```python
from build123d import *

# Parameters (mm, degrees)
SALIENTE_EXTRUIR1_DEPTH = 300
VACIADO1_START          = 47.215476502
VACIADO1_DEPTH          = 295
CROQUIS3_R              = 7.5
CROQUIS3_R_2            = 10
CROQUIS3_W              = 35.4
CROQUIS3_H              = 33.7
CORTAR_EXTRUIR1_DEPTH   = 15
SALIENTE_EXTRUIR2_START = -150
SALIENTE_EXTRUIR2_DEPTH = 150
VACIADO3_START          = 197.215476502
VACIADO3_DEPTH          = 145
CROQUIS5_W              = 5
CROQUIS5_H              = 70
SALIENTE_EXTRUIR3_DEPTH = 145
CROQUIS6_R              = 12.5
CORTAR_EXTRUIR2_DEPTH   = 15
CROQUIS7_W              = 210
CROQUIS7_H              = 255
CORTAR_EXTRUIR3_DEPTH   = 5
SALIENTE_EXTRUIR4_DEPTH = 70
SALIENTE_EXTRUIR5_START = -150
SALIENTE_EXTRUIR5_DEPTH = 150
CORTAR_EXTRUIR6_START   = -150
CORTAR_EXTRUIR6_DEPTH   = 150
CORTAR_EXTRUIR7_START   = -150
CORTAR_EXTRUIR7_DEPTH   = 150
CORTAR_EXTRUIR9_DEPTH   = 15
CROQUIS19_R             = 5
CORTAR_EXTRUIR10_DEPTH  = 15
SALIENTE_EXTRUIR6_START = -5
SALIENTE_EXTRUIR6_DEPTH = 5
CROQUIS21_W             = 25
CROQUIS21_H             = 25
CROQUIS21_R             = 5
SALIENTE_EXTRUIR7_DEPTH = 7
CROQUIS22_R             = 5
CORTAR_EXTRUIR13_DEPTH  = 7
CROQUIS23_W             = 26
CROQUIS23_H             = 24
CROQUIS23_H_2           = 35
CROQUIS23_W_2           = 24
SALIENTE_EXTRUIR8_DEPTH = 20
CROQUIS24_W             = 12
CROQUIS24_H             = 12
CORTAR_EXTRUIR14_DEPTH  = 20


# Read off the part's stored shape, not the designer's step: Vaciado1, Vaciado3
with BuildPart() as part:
    # Croquis2 → Saliente-Extruir1 (new body)
    with BuildSketch(Plane.XY.offset(42.215476502)):
        with BuildLine():
            Line((-130, 55), (130, 55))
            ThreePointArc((130, 55), (124.004556318, -18.45744493), (60, -55))
            Line((60, -55), (-60, -55))
            ThreePointArc((-60, -55), (-124.004556318, -18.45744493), (-130, 55))
        make_face()
    extrude(amount=SALIENTE_EXTRUIR1_DEPTH)

    # Vaciado1 outline → Vaciado1 (cut)
    with BuildSketch(Plane.XY.offset(VACIADO1_START)):
        with BuildLine():
            ThreePointArc((-126.620697254, 50), (-118.915904499, -17.108764781), (-59.914914782, -50))
            Line((-59.914914782, -50), (59.914914782, -50))
            ThreePointArc((59.914914782, -50), (118.915904499, -17.108764781), (126.620697254, 50))
            Line((126.620697254, 50), (-126.620697254, 50))
        make_face()
    extrude(amount=VACIADO1_DEPTH, mode=Mode.SUBTRACT)

    # Croquis3 → Cortar-Extruir1 (cut)
    with BuildSketch(Plane(origin=(0, -55, 0), x_dir=(-1, 0, 0), z_dir=(0, -1, 0))):
        with Locations(Location((30, -178.515476502, 0), (0, 0, 180))):
            Circle(CROQUIS3_R)
        with Locations(Location((0, -178.515476502, 0), (0, 0, 180))):
            Circle(CROQUIS3_R)
        with Locations(Location((-30, -178.515476502, 0), (0, 0, 180))):
            Circle(CROQUIS3_R)
        with Locations(Location((0, -138.515476502, 0), (0, 0, 180))):
            Circle(CROQUIS3_R_2)
        with Locations((0, -225.365476502)):
            Rectangle(CROQUIS3_W, CROQUIS3_H)
    extrude(amount=-CORTAR_EXTRUIR1_DEPTH, mode=Mode.SUBTRACT)

    # Croquis4 → Saliente-Extruir2 (add)
    with BuildSketch(Plane.XY.offset(342.215476502).offset(SALIENTE_EXTRUIR2_START)):
        with BuildLine():
            Line((0, -25), (-112.847078194, -25))
            ThreePointArc((-112.847078194, -25), (-130.13811515, 10.589281798), (-126.620697254, 50))
            Line((-126.620697254, 50), (0, 50))
            Line((0, 50), (126.620697254, 50))
            ThreePointArc((126.620697254, 50), (130.13811515, 10.589281798), (112.847078194, -25))
            Line((112.847078194, -25), (0, -25))
        make_face()
    extrude(amount=SALIENTE_EXTRUIR2_DEPTH)

    # Vaciado3 outline → Vaciado3 (cut)
    with BuildSketch(Plane.XY.offset(VACIADO3_START)):
        with BuildLine():
            Line((126.620697254, 50), (-126.620697254, 50))
            ThreePointArc((-126.620697254, 50), (-130.649934486, 13.762761692), (-116.885919238, -20))
            Line((-116.885919238, -20), (116.885919238, -20))
            ThreePointArc((116.885919238, -20), (130.649934486, 13.762761692), (126.620697254, 50))
        make_face()
    extrude(amount=VACIADO3_DEPTH, mode=Mode.SUBTRACT)

    # Croquis5 → Saliente-Extruir3 (add)
    with BuildSketch(Plane.XY.offset(197.215476502)):
        with Locations((0, 15)):
            Rectangle(CROQUIS5_W, CROQUIS5_H)
    extrude(amount=SALIENTE_EXTRUIR3_DEPTH)

    # Croquis6 → Cortar-Extruir2 (cut)
    with BuildSketch(Plane.XY.offset(197.215476502)):
        with Locations((-62.5, 15)):
            Circle(CROQUIS6_R)
        with Locations((62.5, 15)):
            Circle(CROQUIS6_R)
    extrude(amount=-CORTAR_EXTRUIR2_DEPTH, mode=Mode.SUBTRACT)

    # Croquis7 → Cortar-Extruir3 (cut)
    with BuildSketch(Plane(origin=(0, 55, 0), x_dir=(1, 0, 0), z_dir=(0, 1, 0))):
        with Locations((0, -189.715476502)):
            Rectangle(CROQUIS7_W, CROQUIS7_H)
    extrude(amount=-CORTAR_EXTRUIR3_DEPTH, mode=Mode.SUBTRACT)

    # Croquis8 → Saliente-Extruir4 (add)
    with BuildSketch(Plane(origin=(0, 50, 0), x_dir=(1, 0, 0), z_dir=(0, 1, 0))):
        Polygon((47.439003576, -197.215476502), (2.5, -233.652506429), (2.5, -227.215476502), (39.5, -197.215476502), align=None)
        Polygon((78, -197.215476502), (130, -233.301491229), (130, -227.215476502), (86.769956122, -197.215476502), align=None)
        Polygon((-2.5, -233.652506429), (-47.439003576, -197.215476502), (-39.5, -197.215476502), (-2.5, -227.215476502), align=None)
        Polygon((-78, -197.215476502), (-130, -232.215476502), (-130, -226.188386524), (-86.954533682, -197.215476502), align=None)
    extrude(amount=-SALIENTE_EXTRUIR4_DEPTH)

    # Croquis10 → Saliente-Extruir5 (add)
    with BuildSketch(Plane.XY.offset(342.215476502).offset(SALIENTE_EXTRUIR5_START)):
        with BuildLine():
            Line((-2.5, 45), (-2.5, 50))
            Line((-2.5, 50), (-126.620697254, 50))
            ThreePointArc((-126.620697254, 50), (-127.504866775, 47.514965781), (-128.299912644, 45))
            Line((-128.299912644, 45), (-126.620697254, 45))
            Line((-126.620697254, 45), (-2.5, 45))
        make_face()
        with BuildLine():
            ThreePointArc((128.299912644, 45), (127.504866775, 47.514965781), (126.620697254, 50))
            Line((126.620697254, 50), (2.5, 50))
            Line((2.5, 50), (2.5, 45))
            Line((2.5, 45), (128.299912644, 45))
        make_face()
    extrude(amount=SALIENTE_EXTRUIR5_DEPTH)

    # Croquis13 → Cortar-Extruir6 (cut)
    with BuildSketch(Plane.XY.offset(342.215476502).offset(CORTAR_EXTRUIR6_START)):
        with BuildLine():
            Line((-130, -7.088562093), (-130, -20))
            Line((-130, -20), (-122.997470988, -20))
            ThreePointArc((-122.997470988, -20), (-126.799457266, -13.707377748), (-130, -7.088562093))
        make_face()
    extrude(amount=CORTAR_EXTRUIR6_DEPTH, mode=Mode.SUBTRACT)

    # Croquis14 → Cortar-Extruir7 (cut)
    with BuildSketch(Plane.XY.offset(342.215476502).offset(CORTAR_EXTRUIR7_START)):
        with BuildLine():
            Line((130, -7.088562093), (130, -20))
            Line((130, -20), (122.997470988, -20))
            ThreePointArc((122.997470988, -20), (126.799457266, -13.707377748), (130, -7.088562093))
        make_face()
    extrude(amount=CORTAR_EXTRUIR7_DEPTH, mode=Mode.SUBTRACT)

    # Croquis18 → Cortar-Extruir9 (cut)
    with BuildSketch(Plane(origin=(0, 0, 42.215476502), x_dir=(-1, 0, 0), z_dir=(0, 0, -1))):
        with BuildLine():
            Line((-106.50023103, 50), (106.50023103, 50))
            Line((106.50023103, 50), (106.50023103, 35))
            Line((106.50023103, 35), (125.485042145, 35))
            ThreePointArc((125.485042145, 35), (115.350222936, -15.242927128), (75, -46.848714508))
            Line((75, -46.848714508), (75, -35))
            Line((75, -35), (60, -35))
            Line((60, -35), (60, -50))
            Line((60, -50), (-60, -50))
            Line((-60, -50), (-60, -35))
            Line((-60, -35), (-75, -35))
            Line((-75, -35), (-75, -46.848714508))
            ThreePointArc((-75, -46.848714508), (-115.350222936, -15.242927128), (-125.485042145, 35))
            Line((-125.485042145, 35), (-106.50023103, 35))
            Line((-106.50023103, 35), (-106.50023103, 50))
        make_face()
    extrude(amount=-CORTAR_EXTRUIR9_DEPTH, mode=Mode.SUBTRACT)

    # Croquis19 → Cortar-Extruir10 (cut)
    with BuildSketch(Plane(origin=(0, 0, 42.215476502), x_dir=(-1, 0, 0), z_dir=(0, 0, -1))):
        with Locations((-113.50023103, 42)):
            Circle(CROQUIS19_R)
        with Locations((113.50023103, 42)):
            Circle(CROQUIS19_R)
        with Locations((68, -42)):
            Circle(CROQUIS19_R)
        with Locations((-68, -42)):
            Circle(CROQUIS19_R)
    extrude(amount=-CORTAR_EXTRUIR10_DEPTH, mode=Mode.SUBTRACT)

    # Croquis20 → Saliente-Extruir6 (add)
    with BuildSketch(Plane.XY.offset(342.215476502).offset(SALIENTE_EXTRUIR6_START)):
        with BuildLine():
            Line((112.847078194, -25), (-112.847078194, -25))
            ThreePointArc((-112.847078194, -25), (-88.958164591, -42.956603327), (-59.914914782, -50))
            Line((-59.914914782, -50), (59.914914782, -50))
            ThreePointArc((59.914914782, -50), (88.958164591, -42.956603327), (112.847078194, -25))
        make_face()
    extrude(amount=SALIENTE_EXTRUIR6_DEPTH)

    # Croquis21 → Saliente-Extruir7 (add)
    # profile 1 of 2: a face of its own
    with BuildSketch(Plane(origin=(0, 50, 0), x_dir=(-1, 0, 0), z_dir=(0, -1, 0))):
        with Locations((-102.5, -64.715476502)):
            Rectangle(CROQUIS21_W, CROQUIS21_H)
        with Locations(Location((-98, -69.215476502, 0), (0, 0, 180))):
            Circle(CROQUIS21_R, mode=Mode.SUBTRACT)
    # profile 2 of 2: a face of its own
    with BuildSketch(Plane(origin=(0, 50, 0), x_dir=(-1, 0, 0), z_dir=(0, -1, 0))):
        with Locations((102.5, -64.715476502)):
            Rectangle(CROQUIS21_W, CROQUIS21_H)
        with Locations(Location((98, -69.215476502, 0), (0, 0, 180))):
            Circle(CROQUIS21_R, mode=Mode.SUBTRACT)
    extrude(amount=SALIENTE_EXTRUIR7_DEPTH)

    # Croquis22 → Cortar-Extruir13 (cut)
    with BuildSketch(Plane(origin=(0, 50, 0), x_dir=(1, 0, 0), z_dir=(0, 1, 0))):
        with Locations(Location((-97, -309.215476502, 0), (0, 0, 180))):
            Circle(CROQUIS22_R)
        with Locations(Location((97, -309.215476502, 0), (0, 0, 180))):
            Circle(CROQUIS22_R)
    extrude(amount=-CORTAR_EXTRUIR13_DEPTH, mode=Mode.SUBTRACT)

    # Croquis23 → Saliente-Extruir8 (add)
    with BuildSketch(Plane(origin=(0, -50, 0), x_dir=(1, 0, 0), z_dir=(0, 1, 0))):
        Polygon((18, -161.515476502), (18, -121.515476502), (-17, -121.515476502), (-17, -161.515476502), (-47, -161.515476502), (-47, -195.515476502), (47, -195.515476502), (47, -161.515476502), align=None)
        with Locations((29, -178.515476502)):
            Rectangle(CROQUIS23_W, CROQUIS23_H, mode=Mode.SUBTRACT)
        with Locations((-29, -178.515476502)):
            Rectangle(CROQUIS23_W, CROQUIS23_H, mode=Mode.SUBTRACT)
        with Locations((0, -144.015476502)):
            Rectangle(CROQUIS23_W, CROQUIS23_H_2, mode=Mode.SUBTRACT)
        with Locations((0, -178.515476502)):
            Rectangle(CROQUIS23_W_2, CROQUIS23_H, mode=Mode.SUBTRACT)
    extrude(amount=SALIENTE_EXTRUIR8_DEPTH)

    # Croquis24 → Cortar-Extruir14 (cut)
    with BuildSketch(Plane(origin=(0, 50, 0), x_dir=(1, 0, 0), z_dir=(0, 1, 0))):
        with Locations((62.719501788, -213.215476502)):
            Rectangle(CROQUIS24_W, CROQUIS24_H)
        with Locations((-62.719501788, -213.215476502)):
            Rectangle(CROQUIS24_W, CROQUIS24_H)
    extrude(amount=-CORTAR_EXTRUIR14_DEPTH, mode=Mode.SUBTRACT)


solid = part.part
```
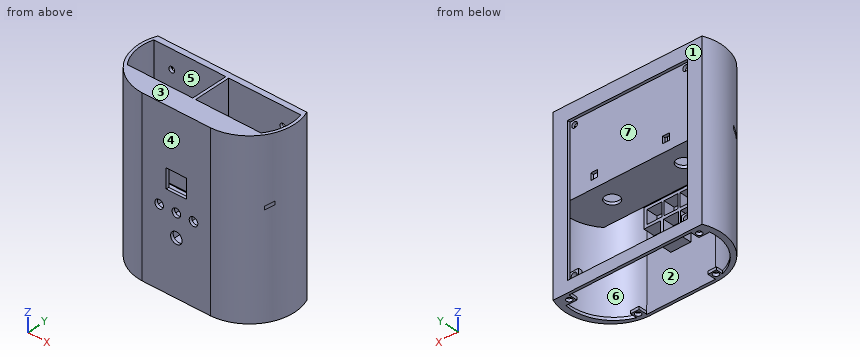
Here's how the part is built. I have some questions about the finished solid (model axes, mm). Face numbers are marked on the shaded views. A direction names the side the tool comes from. Coordinates: 2 decimals unless noted, no trailing zeros. Loops run counter-clockwise (first coordinate to the right, second up) from the corner with the lowest first, then second, coordinate; pieces in that order, holes last. Notation, with made-up numbers: (-24.75, 26) - (-20.75, 26) arc R34 ccw to (-20.75, 64) - close; hole circle Ø5 at (40.25, 84). An arc over 180 degrees is marked (long way). Answer as CSV lines item,"result".
Q1. For the marked faces 4, 5, 6 and 7, which set-ups out of +Z, -Z, +X, -X, +Y, -Y let a thin tool reach every point of the face, with its end or its side?
Response:
face 4,"+Z, -Z, +X, -X, -Y"
face 5,"+Z"
face 6,"none"
face 7,"+Y"
Q2. We'd pull the mould along Z, two halves only. Please class the marked faces 1, 2 and 3: pulls with the +Z half, pulls with the -Z half, needs draft (parallel to the pull), parting line crosses it, or undercut.
Response:
face 1,"needs draft"
face 2,"undercut"
face 3,"pulls with the +Z half"
Q3. If I drill on L1, parallel to Y at x = -38, z = 326; L2, parallel to Z at x = 14, y = -49; L3, parallel to Y at x = -52, z = 271, over which ranges is the centre line in solid material (lowest first)? Write a range as [from, to].
Response:
L1,"[-55, -50], [-25, -20], [45, 55]"
L2,"[121.52, 195.52], [337.22, 342.22]"
L3,"[-55, -50], [-25, -20], [45, 50]"
Q4. If we section it at B-B, the plane x = 30: Give the number of separate pieces and of enclosed holes in the cut face, and give its area (3 significant figures).
Response:
separate pieces,"3"
enclosed holes,"1"
area,"4,220 mm2"
Q5. If we section it at A-A, the plane z = 105: Write out the boundary of the cut face in (x, y).
Response:
outline,"(-130, 55) arc R79 ccw to (-60, -55) - (60, -55) arc R79 ccw to (130, 55) - (105, 55) - (105, 50) - (126.62, 50) arc R74 cw to (59.91, -50) - (-59.91, -50) arc R74 cw to (-126.62, 50) - (-105, 50) - (-105, 55) - close"
Q6. If we section it at C-C, the plane z = 271.5: Write out the boundary of the cut face in (x, y).
Response:
outline,"(-130, 55) arc R79 ccw to (-60, -55) - (60, -55) arc R79 ccw to (130, 55) - (105, 55) - (105, 50) - (-105, 50) - (-105, 55) - close; hole (-128.3, 45) arc R74 ccw to (-116.89, -20) - (-2.5, -20) - (-2.5, 45) - close; hole (-112.85, -25) arc R74 ccw to (-59.91, -50) - (59.91, -50) arc R74 ccw to (112.85, -25) - close; hole (2.5, -20) - (116.89, -20) arc R74 ccw to (128.3, 45) - (2.5, 45) - close"
Q7. For pin 1 (6 mm diameter, centred on y = -40, z = 270, fed in from -X); pin 2 (7.5 mm diameter, centred on x = 99, z = 69.5, fed in from +Y) (3 decimals); pin 3 (2.5 mm diameter, centred on y = 48, z = 211, fed in from -X), each with a flat end and sliding along its axis, tell me the tip position at first contact or that it passes through.
Response:
pin 1,"x = -107.61"
pin 2,"y = -34.485"
pin 3,"x = -133"
